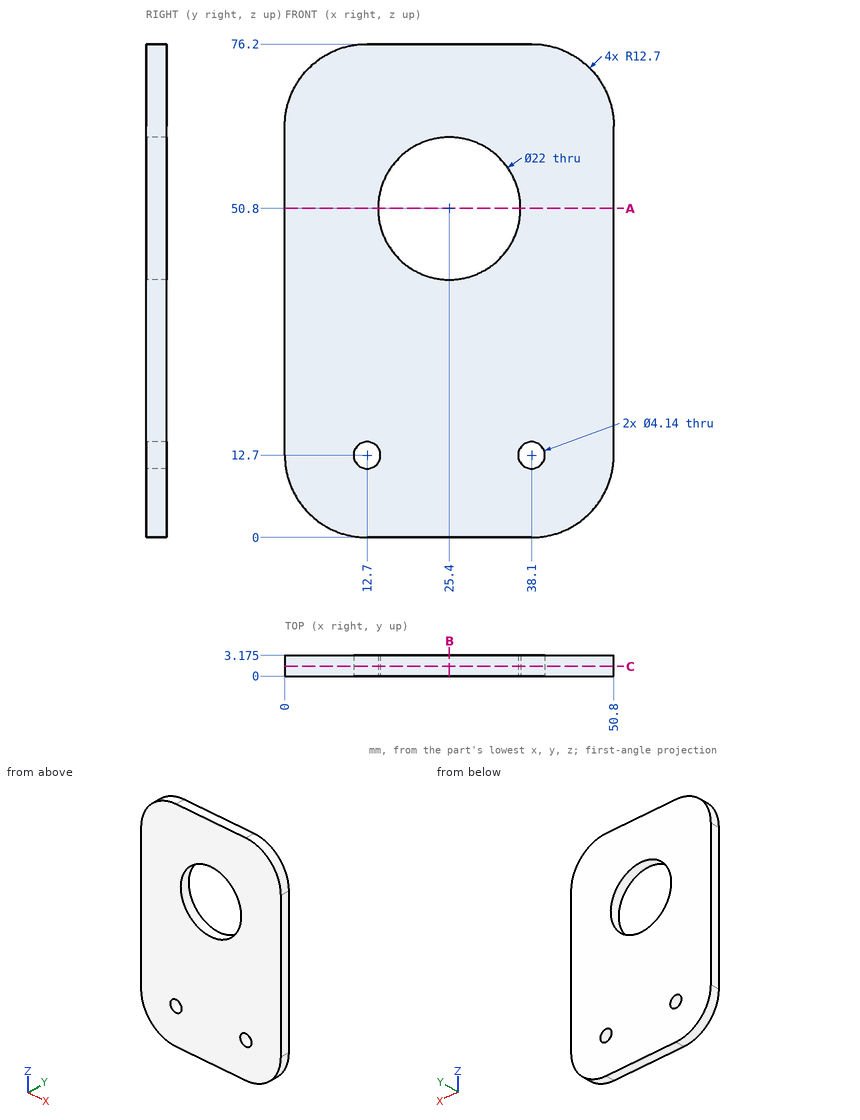
Can you work these out from the drawing? Everything is in mm from the part's minimum corner. Coordinates: 2 decimals unless noted, no trailing zeros. Write each loop counter-clockwise with the first axis right and the second up, starting at its lowest first coordinate (ties: lowest second). Pieces come first, ordered by that corner, then holes. Notation, with made-up numbers: (-35, -20) -> (-31, -20) arc R26 cw to (-31, 14) -> close; hole circle Ø11 at (88.25, -7). An arc over 180 degrees is marked (long way). Write each question's results on one line, items separated by ' | '. Start each with the question number.
Item 1: Please list where these lines run through material, in increasing order: probe 1 along X at (y, z) = (0.95, 12.7); probe 2 along Z at (x, y) = (25.4, 1.85); probe 3 along Z at (x, y) = (12.7, 2.3).
Item 2: If we section it at C-C, the plane y = 1.5: Write out the boundary of the cut face in (x, z), and give its area (3 significant figures).
Item 3: If we section it at A-A, the plane z = 50.8: Write out the boundary of the cut face in (x, y) (3 decimals).
Item 4: I'm going to push flat-ended pins straight in: P1, Ø8, axis at x = 27.5, z = 56.5, coming from the +Y side; P2, Ø12, axis at x = 16.5, z = 41.5, coming from the -Y side. Where does each tip first touch, or does it pass through?
Item 5: If we section it at B-B, the plane x = 25.4: Write out the boundary of the cut face in (y, z) (3 decimals).
Answer block:
1) probe 1: 0 to 10.63, 14.77 to 36.03, 40.17 to 50.8 | probe 2: 0 to 39.8, 61.8 to 76.2 | probe 3: 0 to 10.63, 14.77 to 76.2
2) outline: (0, 12.7) arc R12.7 ccw to (12.7, 0) -> (38.1, 0) arc R12.7 ccw to (50.8, 12.7) -> (50.8, 63.5) arc R12.7 ccw to (38.1, 76.2) -> (12.7, 76.2) arc R12.7 ccw to (0, 63.5) -> close; hole circle Ø4.14 at (12.7, 12.7); hole circle Ø22 at (25.4, 50.8); hole circle Ø4.14 at (38.1, 12.7) | area: 3,330 mm²
3) outline: (0, 0) -> (14.4, 0) -> (14.4, 3.175) -> (0, 3.175) -> close; (36.4, 0) -> (50.8, 0) -> (50.8, 3.175) -> (36.4, 3.175) -> close
4) P1: through | P2: y = 0
5) outline: (0, 0) -> (3.175, 0) -> (3.175, 39.8) -> (0, 39.8) -> close; (0, 61.8) -> (3.175, 61.8) -> (3.175, 76.2) -> (0, 76.2) -> close
